```python
from build123d import *

# Parameters (mm, degrees)
F0_W     = 30
F0_H     = 29
F0_R     = 2
F0_R_2   = 5
F1_DEPTH = 4
F2_R     = 4
F3_SIZE  = 2


with BuildPart() as f1:
    # F0 (on Top) → F1 (new body)
    with BuildSketch(Plane.XY):
        with Locations((0, -0.5)):
            Rectangle(F0_W, F0_H)
        with Locations((-11, -10)):
            Circle(F0_R, mode=Mode.SUBTRACT)
        with Locations((11, -10)):
            Circle(F0_R, mode=Mode.SUBTRACT)
        with Locations((-11, 10)):
            Circle(F0_R, mode=Mode.SUBTRACT)
        Circle(F0_R_2, mode=Mode.SUBTRACT)
        with Locations((11, 10)):
            Circle(F0_R, mode=Mode.SUBTRACT)
    extrude(amount=F1_DEPTH)

    # F2
    f2_edges = [f1.edges().sort_by_distance(p)[0] for p in [
        (-15, 14, 2),
        (15, 14, 2),
        (-15, -15, 2),
        (15, -15, 2),
    ]]
    fillet(f2_edges, radius=F2_R)

    # F3
    f3_edges = [f1.edges().sort_by_distance(p)[0] for p in [
        (-5, 0, 4),
    ]]
    chamfer(f3_edges, length=F3_SIZE)


solid = f1.part
```
Model file for the job. Use its own axes, mm. Give positions to 0.01 mm unless a question says otherwise; leave off trailing zeros. Order: outer loops, then holes, each group sorted by start corner. A loop starts at its lowest first (then second) coordinate and runs counter-clockwise, first axis right, second up.
1) Mould opens along X. For faces 1 (the cylindrical face through (13.797, -13.859, 2.028)), 2 (the flat face through (-15, -1, 2)), 3 (the cylindrical face through (9.526, 11.352, 1.972)) say: +X half, -X half, draft (parallel to the pull), parting line (faces both ways), or undercut.
2) Saw through at B-B, the plane z = 0.65. Write the cut outline in (x, y), then the cut area to 3 significant figures.
3) Saw through at D-D, the plane y = -10. Write the cut outline in (x, z), then the cut area to 3 significant figures.
4) Wall check: probe 1 along Y at (x, z) = (11, 1.9); probe 2 along Y at (x, z) = (-11.5, 3.1); probe 3 along X at (y, z) = (10.5, 1.15). Give the ranges that are in metal, low to high.
5) Saw through at A-A, the plane y = 0. Write the cut outline in (x, z).
6) Pin check, flat tip, straight feed: pin 1 (13 mm diameter, centred on x = 0, y = 0, fed in from +Z). Stop position of the tip, or through.
7) Saw through at C-C, the plane x = 0. Write the cut outline in (y, z), then the cut area to 3 significant figures.
Computed:
1. face 1: +X half
1. face 2: -X half
1. face 3: undercut
2. outline: (-15, -11) arc R4 ccw to (-11, -15) - (11, -15) arc R4 ccw to (15, -11) - (15, 10) arc R4 ccw to (11, 14) - (-11, 14) arc R4 ccw to (-15, 10) - close; hole circle Ø4 at (-11, -10); hole circle Ø4 at (-11, 10); hole circle Ø10 at (0, 0); hole circle Ø4 at (11, -10); hole circle Ø4 at (11, 10)
2. area: 727 mm2
3. outline: (-15, 0) - (-13, 0) - (-13, 4) - (-15, 4) - close; (-9, 0) - (9, 0) - (9, 4) - (-9, 4) - close; (13, 0) - (15, 0) - (15, 4) - (13, 4) - close
3. area: 88.0 mm2
4. probe 1: y = -15 to -12, -8 to 8, 12 to 14
4. probe 2: y = -14.97 to -11.94, -8.06 to 8.06, 11.94 to 13.97
4. probe 3: x = -14.97 to -12.94, -9.06 to 9.06, 12.94 to 14.97
5. outline: (-15, 0) - (-5, 0) - (-5, 2) - (-7, 4) - (-15, 4) - close; (5, 0) - (15, 0) - (15, 4) - (7, 4) - (5, 2) - close
6. pin 1: stops at z = 3.5
7. outline: (-15, 0) - (-5, 0) - (-5, 2) - (-7, 4) - (-15, 4) - close; (5, 0) - (14, 0) - (14, 4) - (7, 4) - (5, 2) - close
7. area: 72.0 mm2
